CAD build for the part. Positions are in the model's coordinates, mm. A direction names the side the tool comes from. Give positions to 0.01 mm unless a question says otherwise; leave off trailing zeros. Order: outer loops, then holes, each group sorted by start corner. A loop starts at its lowest first (then second) coordinate and runs counter-clockwise, first axis right, second up.
Item 1: Which spindle directions (+Z, -Z, +X, -X, +Y, -Y) get a long thin tool onto all of the face, cutting with end or side? Do faces 1 (the flat face through (68, 88.9, 38)), 2 (the cylindrical face through (-60.47, -76.378, -46.367)), 3 (the flat face through (16, 63.5, 1)). Say none if no direction does.
Item 2: Band-saw the part on B-B on z = 0. Give the cut face in (x, y).
Item 3: Band-saw the part on A-A on x = 0. Give the cut face in (y, z), plus the area to 3 significant figures.
Item 4: Flat gauge pins, fed straight in: P1, Ø12, axis at y = 31.5, z = 117, coming from the +X side; P2, Ø18.5, axis at x = 0, z = 0, coming from the +Y side; P3, Ø4, axis at x = 111.5, y = -13, coming from the +Z side. Where does each tip first touch, or does it go through?
Item 5: Two-plate mould, pull along Z, no slides. Class faces 4 (the flat face through (68, -88.9, 38)), 5 (the flat face through (16, -63.5, 1)), 6 (the cylindrical face through (-1.72, -0.89, -7.75)), 7 (the cylindrical face through (-146.1, -0.9, -112.1)): released by +Z, released by -Z, zero draft, split by the parting line, or undercut.
Item 6: Wall check: L1, parallel to Y at x = 55, z = 15.5; L2, parallel to Z at x = 0, y = -80.75; L3, parallel to Z at x = 0, y = 78.25. Give the ranges that are in metal, low to high.
```python
from build123d import *

# Parameters (mm, degrees)
F0_R      = 184.15
F1_DEPTH  = 88.9
F2_R      = 76.2
F3_DEPTH  = 25.4
F4_R      = 76.2
F5_DEPTH  = 25.4
F6_R      = 12.7
F7_DEPTH  = 177.8
F8_R      = 25.4
F9_R      = 12.7
F9_R_2    = 7.9375
F10_DEPTH = 127


with BuildPart() as f1:
    # F0 (on Front) → F1 (new body, symmetric)
    with BuildSketch(Plane.XZ):
        Circle(F0_R)
    extrude(amount=F1_DEPTH, both=True)

    # F2 (on face) → F3 (cut)
    with BuildSketch(Plane.XZ.offset(88.9)):
        Circle(F2_R)
    extrude(amount=-F3_DEPTH, mode=Mode.SUBTRACT)

    # F4 (on face) → F5 (cut)
    with BuildSketch(Plane(origin=(0, 88.9, 0), x_dir=(-1, 0, 0), z_dir=(0, 1, 0))):
        Circle(F4_R)
    extrude(amount=-F5_DEPTH, mode=Mode.SUBTRACT)

    # F6 (on face) → F7 (cut, symmetric)
    with BuildSketch(Plane.XZ.offset(88.9)):
        Circle(F6_R)
    extrude(amount=F7_DEPTH, both=True, mode=Mode.SUBTRACT)

    # F8
    f8_edges = [f1.edges().sort_by_distance(p)[0] for p in [
        (-184.15, 88.9, 0),
        (-184.15, -88.9, 0),
    ]]
    fillet(f8_edges, radius=F8_R)

    # F9 (on face) → F10 (join)
    with BuildSketch(Plane.XZ.offset(63.5)):
        Circle(F9_R)
        Circle(F9_R_2, mode=Mode.SUBTRACT)
    extrude(amount=-F10_DEPTH)


solid = f1.part
```
The answers:
1. face 1: +Z, -Z, +X, -X, +Y
1. face 2: -Y
1. face 3: +Y
2. outline: (-184.15, -63.5) arc R25.4 ccw to (-158.75, -88.9) - (-76.2, -88.9) - (-76.2, -63.5) - (-7.94, -63.5) - (-7.94, 63.5) - (-76.2, 63.5) - (-76.2, 88.9) - (-158.75, 88.9) arc R25.4 ccw to (-184.15, 63.5) - close; (7.94, -63.5) - (76.2, -63.5) - (76.2, -88.9) - (158.75, -88.9) arc R25.4 ccw to (184.15, -63.5) - (184.15, 63.5) arc R25.4 ccw to (158.75, 88.9) - (76.2, 88.9) - (76.2, 63.5) - (7.94, 63.5) - close
3. outline: (-88.9, -158.75) arc R25.4 ccw to (-63.5, -184.15) - (63.5, -184.15) arc R25.4 ccw to (88.9, -158.75) - (88.9, -76.2) - (63.5, -76.2) - (63.5, -7.94) - (-63.5, -7.94) - (-63.5, -76.2) - (-88.9, -76.2) - close; (-88.9, 76.2) - (-63.5, 76.2) - (-63.5, 7.94) - (63.5, 7.94) - (63.5, 76.2) - (88.9, 76.2) - (88.9, 158.75) arc R25.4 ccw to (63.5, 184.15) - (-63.5, 184.15) arc R25.4 ccw to (-88.9, 158.75) - close
3. area: 55,200 mm2
4. P1: stops at x = 146.94
4. P2: stops at y = 63.5
4. P3: stops at z = 148.06
5. face 4: zero draft
5. face 5: undercut
5. face 6: undercut
5. face 7: split by the parting line
6. L1: y = -63.5 to 63.5
6. L2: z = -177.39 to -76.2, 76.2 to 177.39
6. L3: z = -179.43 to -76.2, 76.2 to 179.43
